Can you work these out from the model? Positions are in its coordinate system, mm. A direction names the side the tool comes from. Give positions to 0.01 mm unless a question says otherwise; leave off trailing zeros. Loops run counter-clockwise (first coordinate to the right, second up) from the corner with the lowest first, then second, coordinate; pieces in that order, holes last. Notation, with made-up numbers: (5, 18.5) -> (10, 18.5) arc R32 cw to (10, 47.5) -> close; hole circle Ø2 at (51, 27.25). An arc over 180 degrees is marked (long way). Use CSV: the item, a comma, the result in double quotes.
from build123d import *

# Parameters (mm, degrees)
SKETCH1_R               = 50
BOSS_EXTRUDE1_DEPTH     = 250
BOSS_EXTRUDE2_DEPTH     = 55
SKETCH7_R               = 1.25
CUT_EXTRUDE4_DEPTH      = 75
CUT_EXTRUDE4_DEPTH_BACK = 96
CUT_EXTRUDE5_DEPTH      = 96
CUT_EXTRUDE6_DEPTH      = 96
SKETCH10_R              = 1.25
CUT_EXTRUDE7_DEPTH      = 96


with BuildPart() as part:
    # Sketch1 → Boss-Extrude1 (new body)
    with BuildSketch(Plane.XY):
        Circle(SKETCH1_R)
        with BuildLine():
            Line((-44.955555556, 1.999506112), (-47.255555556, 1.999506112))
            Line((-47.255555556, 1.999506112), (-47.255555556, -1.999506112))
            Line((-47.255555556, -1.999506112), (-44.955555556, -1.999506112))
            ThreePointArc((-44.955555556, -1.999506112), (0, -45), (44.955555556, -1.999506112))
            Line((44.955555556, -1.999506112), (47.255555556, -1.999506112))
            Line((47.255555556, -1.999506112), (47.255555556, 1.999506112))
            Line((47.255555556, 1.999506112), (44.955555556, 1.999506112))
            ThreePointArc((44.955555556, 1.999506112), (0, 45), (-44.955555556, 1.999506112))
        make_face(mode=Mode.SUBTRACT)
    extrude(amount=BOSS_EXTRUDE1_DEPTH)

    # Sketch3 → Boss-Extrude2 (add)
    with BuildSketch(Plane.XY.offset(250)):
        Polygon((28.2, 0), (28.2, 35.067934071), (35.640426485, 35.067934071), (35.640426485, -35.067934071), (28.2, -35.067934071), align=None)
    extrude(amount=BOSS_EXTRUDE2_DEPTH)

    # Sketch7 → Cut-Extrude4 (cut, two sides)
    with BuildSketch(Plane(origin=(35.640426485, 0, 0), x_dir=(0, 0, -1), z_dir=(1, 0, 0))) as cut_extrude4_sk:
        with Locations((-100, 0)):
            Circle(SKETCH7_R)
    extrude(amount=CUT_EXTRUDE4_DEPTH, mode=Mode.SUBTRACT)
    extrude(cut_extrude4_sk.sketch, amount=-CUT_EXTRUDE4_DEPTH_BACK, mode=Mode.SUBTRACT)

    # Sketch8 → Cut-Extrude5 (cut)
    with BuildSketch(Plane(origin=(35.640426485, 0, 0), x_dir=(0, 0, -1), z_dir=(1, 0, 0))):
        with BuildLine():
            Line((-287.5, 17.5), (-250, 35.067934071))
            Line((-250, 35.067934071), (-305, 35.067934071))
            Line((-305, 35.067934071), (-305, 0))
            ThreePointArc((-305, 0), (-299.874368671, 12.374368671), (-287.5, 17.5))
        make_face()
    extrude(amount=-CUT_EXTRUDE5_DEPTH, mode=Mode.SUBTRACT)

    # Sketch9 → Cut-Extrude6 (cut)
    with BuildSketch(Plane(origin=(35.640426485, 0, 0), x_dir=(0, 0, -1), z_dir=(1, 0, 0))):
        with BuildLine():
            Line((-287.5, -17.5), (-250, -35.067934071))
            Line((-250, -35.067934071), (-305, -35.067934071))
            Line((-305, -35.067934071), (-305, 0))
            ThreePointArc((-305, 0), (-299.874368671, -12.374368671), (-287.5, -17.5))
        make_face()
    extrude(amount=-CUT_EXTRUDE6_DEPTH, mode=Mode.SUBTRACT)

    # Sketch10 → Cut-Extrude7 (cut)
    with BuildSketch(Plane(origin=(35.640426485, 0, 0), x_dir=(0, 0, -1), z_dir=(1, 0, 0))):
        with Locations((-296.25, 0)):
            Circle(SKETCH10_R)
        with Locations((-287.5, 8.75)):
            Circle(SKETCH10_R)
        with Locations((-278.75, 0)):
            Circle(SKETCH10_R)
        with Locations((-287.5, -8.75)):
            Circle(SKETCH10_R)
    extrude(amount=-CUT_EXTRUDE7_DEPTH, mode=Mode.SUBTRACT)


solid = part.part
(1) If I drill on L1, parallel to Y at x = 31.25, z = 287.5; L2, parallel to Z at x = 48, y = 0; L3, parallel to X at y = -8, z = 278, over which ranges is the centre line in solid material (lowest first)? Write a range as from..to.
Answer sheet:
L1,"y = -17.5..-10, -7.5..7.5, 10..17.5"
L2,"z = 0..98.75, 101.25..250"
L3,"x = 28.2..35.64"
(2) Will these pins go through, and if not, where does the flat tip stop? pin 1 Ø1 at (y, z) = (-21, 197) entering from -X; pin 2 Ø1.1 at (x, z) = (46, 182) entering from -Y; pin 3 Ø2.5 at (x, z) = (46, 117) entering from +Y.
Answer sheet:
pin 1,"stops at x = -45.6"
pin 2,"stops at y = -20.84"
pin 3,"stops at y = 22.3"
(3) If we section it at B-B, the plane x = 13: Write out the boundary of the cut face in (y, z).
Answer sheet:
outline,"(-48.28, 0) -> (-43.08, 0) -> (-43.08, 250) -> (-48.28, 250) -> close; (43.08, 0) -> (48.28, 0) -> (48.28, 250) -> (43.08, 250) -> close"
(4) If we section it at C-C, the plane y = -32: Write out the boundary of the cut face in (x, z), then the cut area to 3 significant figures.
Answer sheet:
outline,"(-38.42, 0) -> (-31.64, 0) -> (-31.64, 250) -> (-38.42, 250) -> close; (28.2, 250) -> (31.64, 250) -> (31.64, 0) -> (38.42, 0) -> (38.42, 250) -> (35.64, 250) -> (35.64, 256.55) -> (28.2, 256.55) -> close"
area,"3,440 mm2"
(5) If we section it at D-D, the plane y = -13.5: Write out the boundary of the cut face in (x, z), then the cut area to 3 significant figures.
Answer sheet:
outline,"(-48.14, 0) -> (-42.93, 0) -> (-42.93, 250) -> (-48.14, 250) -> close; (28.2, 250) -> (35.64, 250) -> (35.64, 298.64) -> (28.2, 298.64) -> close; (42.93, 0) -> (48.14, 0) -> (48.14, 250) -> (42.93, 250) -> close"
area,"2,970 mm2"
(6) Which directions (+Z, -Z, +X, -X, +Y, -Y) give clear straight access to the entire face, cutting with the end or side of a thin tool? Please do faces 1 (the face through (45.4, 2.8, 250)), 2 (the face through (32, 0, 250)), 3 (the face through (31.97, 26.16, 269.01)).
Answer sheet:
face 1,"+Z, +X, +Y, -Y"
face 2,"-Z"
face 3,"+Z, +X, -X, +Y"
(7) We'd pull the mould along Y, two halves only. Please class faces 4 (the face through (31.97, -26.16, 269.01)), 5 (the face through (-0.96, -44.99, 123.25)), 6 (the face through (28.2, 0, 271)), 7 (the face through (47.69, 15.02, 123.25)): released by +Y, released by -Y, zero draft, split by the parting line, or undercut.
Answer sheet:
face 4,"released by -Y"
face 5,"undercut"
face 6,"zero draft"
face 7,"split by the parting line"
